Could you check a few things on this model? Use its own coordinates, in mm. Give positions to 0.01 mm unless a question says otherwise; leave off trailing zeros. Answer as CSV lines item,"result". Start each with the question number.
Q1. Will these pins go through, and if not, where does the flat tip stop? pin 1 Ø1.2 at (x, z) = (178, 2.5) entering from +Y; pin 2 Ø0.5 at (x, y) = (145.5, 14) entering from -Z; pin 3 Ø1.4 at (x, z) = (190, 14) entering from +Y.
Q2. If I drill on line 1 along Z through (x, y) = (228.5, 11.5); line 2 along Z through (x, y) = (40, 12.5); line 3 along Z through (x, y) = (79, 0), over which ranges is the centre line in solid material (lowest first)?
Q3. Imagine slicing it at A-A on x = 95.5. State how many separate pieces and enclosed holes the cut face has, and give its area (3 significant figures).
Q4. We'd pull the mould along Y, two halves only. Please class faces 1 (the face through (148, 15, -9)), 2 (the face through (148, -15, -9)), 3 (the face through (147.9, -0.74, -3.32)), 4 (the face through (0, -4, 0)): pulls with the +Y half, pulls with the -Y half, needs draft (parallel to the pull), parting line crosses it, or undercut.
```python
from build123d import *

# Parameters (mm, degrees)
SKETCH_1_R              = 2.1
SKETCH_1_R_2            = 3.4
F_30XS6_30X30S6_1_DEPTH = 300


with BuildPart() as part:
    # 草图1 → 30xs6 30X30S6(1) (new body)
    with BuildSketch(Plane.YZ):
        with BuildLine():
            Line((-14.7, 4), (-13, 4))
            Line((-13, 4), (-13, 8.25))
            Line((-13, 8.25), (-9.664213562, 8.25))
            Line((-9.664213562, 8.25), (-6, 4.585786438))
            Line((-6, 4.585786438), (-6, 0.519615242))
            Line((-6, 0.519615242), (-5.7, 0))
            Line((-5.7, 0), (-6, -0.519615242))
            Line((-6, -0.519615242), (-6, -4.585786438))
            Line((-6, -4.585786438), (-9.664213562, -8.25))
            Line((-9.664213562, -8.25), (-13, -8.25))
            Line((-13, -8.25), (-13, -4))
            Line((-13, -4), (-14.7, -4))
            ThreePointArc((-14.7, -4), (-14.912132034, -4.087867966), (-15, -4.3))
            Line((-15, -4.3), (-15, -13))
            ThreePointArc((-15, -13), (-14.414213562, -14.414213562), (-13, -15))
            Line((-13, -15), (-4.3, -15))
            ThreePointArc((-4.3, -15), (-4.087867966, -14.912132034), (-4, -14.7))
            Line((-4, -14.7), (-4, -13))
            Line((-4, -13), (-8.25, -13))
            Line((-8.25, -13), (-8.25, -9.664213562))
            Line((-8.25, -9.664213562), (-4.585786438, -6))
            Line((-4.585786438, -6), (-0.519615242, -6))
            Line((-0.519615242, -6), (0, -5.7))
            Line((0, -5.7), (0.519615242, -6))
            Line((0.519615242, -6), (4.585786438, -6))
            Line((4.585786438, -6), (8.25, -9.664213562))
            Line((8.25, -9.664213562), (8.25, -13))
            Line((8.25, -13), (4, -13))
            Line((4, -13), (4, -14.7))
            ThreePointArc((4, -14.7), (4.087867966, -14.912132034), (4.3, -15))
            Line((4.3, -15), (13, -15))
            ThreePointArc((13, -15), (14.414213562, -14.414213562), (15, -13))
            Line((15, -13), (15, -4.3))
            ThreePointArc((15, -4.3), (14.912132034, -4.087867966), (14.7, -4))
            Line((14.7, -4), (13, -4))
            Line((13, -4), (13, -8.25))
            Line((13, -8.25), (9.664213562, -8.25))
            Line((9.664213562, -8.25), (6, -4.585786438))
            Line((6, -4.585786438), (6, -0.519615242))
            Line((6, -0.519615242), (5.7, 0))
            Line((5.7, 0), (6, 0.519615242))
            Line((6, 0.519615242), (6, 4.585786438))
            Line((6, 4.585786438), (9.664213562, 8.25))
            Line((9.664213562, 8.25), (13, 8.25))
            Line((13, 8.25), (13, 4))
            Line((13, 4), (14.7, 4))
            ThreePointArc((14.7, 4), (14.912132034, 4.087867966), (15, 4.3))
            Line((15, 4.3), (15, 13))
            ThreePointArc((15, 13), (14.414213562, 14.414213562), (13, 15))
            Line((13, 15), (4.3, 15))
            ThreePointArc((4.3, 15), (4.087867966, 14.912132034), (4, 14.7))
            Line((4, 14.7), (4, 13))
            Line((4, 13), (8.25, 13))
            Line((8.25, 13), (8.25, 9.664213562))
            Line((8.25, 9.664213562), (4.585786438, 6))
            Line((4.585786438, 6), (0.519615242, 6))
            Line((0.519615242, 6), (0, 5.7))
            Line((0, 5.7), (-0.519615242, 6))
            Line((-0.519615242, 6), (-4.585786438, 6))
            Line((-4.585786438, 6), (-8.25, 9.664213562))
            Line((-8.25, 9.664213562), (-8.25, 13))
            Line((-8.25, 13), (-4, 13))
            Line((-4, 13), (-4, 14.7))
            ThreePointArc((-4, 14.7), (-4.087867966, 14.912132034), (-4.3, 15))
            Line((-4.3, 15), (-13, 15))
            ThreePointArc((-13, 15), (-14.414213562, 14.414213562), (-15, 13))
            Line((-15, 13), (-15, 4.3))
            ThreePointArc((-15, 4.3), (-14.912132034, 4.087867966), (-14.7, 4))
        make_face()
        with Locations((11.625, 11.625)):
            Circle(SKETCH_1_R, mode=Mode.SUBTRACT)
        with Locations((11.625, -11.625)):
            Circle(SKETCH_1_R, mode=Mode.SUBTRACT)
        Circle(SKETCH_1_R_2, mode=Mode.SUBTRACT)
        with Locations((-11.625, -11.625)):
            Circle(SKETCH_1_R, mode=Mode.SUBTRACT)
        with Locations((-11.625, 11.625)):
            Circle(SKETCH_1_R, mode=Mode.SUBTRACT)
    extrude(amount=F_30XS6_30X30S6_1_DEPTH)


solid = part.part
```
Conclusion:
1,pin 1,"y = 6"
1,pin 2,"z = -14.85"
1,pin 3,"y = 14.98"
2,line 1,"-15 to -13.72, -9.53 to -8.25, 8.25 to 9.53, 13.72 to 15"
2,line 2,"-15 to -13.53, -9.72 to -8.25, 8.25 to 9.72, 13.53 to 15"
2,line 3,"-5.7 to -3.4, 3.4 to 5.7"
3,separate pieces,"1"
3,enclosed holes,"5"
3,area,"332 mm^2"
4,face 1,"pulls with the +Y half"
4,face 2,"pulls with the -Y half"
4,face 3,"undercut"
4,face 4,"needs draft"
